Build history of the part. All positions in model axes, mm. Face numbers are marked on the shaded views. A direction names the side the tool comes from. Coordinates: 2 decimals unless noted, no trailing zeros. Loops run counter-clockwise (first coordinate to the right, second up) from the corner with the lowest first, then second, coordinate; pieces in that order, holes last. Notation, with made-up numbers: (-34, 63) - (-1, 63) arc R30 ccw to (-1, 100) - close; hole circle Ø11 at (42.25, 76.5). An arc over 180 degrees is marked (long way). One line per item, written item: value.
```python
from build123d import *

# Parameters (mm, degrees)
SKETCH001_W  = 6
SKETCH001_H  = 6
PAD001_DEPTH = 0.1
FILLET001_R  = 0.3
PAD008_DEPTH = 0.7
FILLET003_R  = 0.29
PAD009_DEPTH = 0.7
FILLET004_R  = 0.29
PAD010_DEPTH = 0.7
FILLET005_R  = 0.29
SKETCH_W     = 6
SKETCH_H     = 6
PAD_DEPTH    = 3.5
FILLET_R     = 0.3
SKETCH004_R  = 0.5
PAD003_DEPTH = 0.6
SKETCH003_R  = 0.5
PAD004_DEPTH = 0.6
SKETCH005_R  = 0.5
PAD002_DEPTH = 0.6
SKETCH002_R  = 0.5
PAD005_DEPTH = 0.6
SKETCH006_R  = 1.75
PAD006_DEPTH = 1.5
FILLET006_R  = 0.1
PAD007_DEPTH = 0.7
FILLET002_R  = 0.29


with BuildPart() as fillet001:
    # Sketch001 → Pad001 (new body)
    with BuildSketch(Plane.XY.offset(3.5)):
        with Locations((3.15, -2.25)):
            Rectangle(SKETCH001_W, SKETCH001_H)
    extrude(amount=PAD001_DEPTH)

    # Fillet001
    fillet001_edges = [fillet001.edges().sort_by_distance(p)[0] for p in [
        (6.15, -5.25, 3.55),
        (0.15, -5.25, 3.55),
        (6.15, 0.75, 3.55),
        (0.15, 0.75, 3.55),
    ]]
    fillet(fillet001_edges, radius=FILLET001_R)


with BuildPart() as fillet003:
    # Sketch008 → Pad008 (new body)
    with BuildSketch(Plane.XZ.offset(0.35)):
        Polygon((-0.15, 1.5), (0.15, 1.5), (0.15, -0.5), (-0.15, -1.5), (0.15, -2.5), (0.15, -3.5), (-0.15, -3.5), (-0.15, -2.5), (-0.45, -1.5), (-0.15, -0.5), align=None)
    extrude(amount=-PAD008_DEPTH)

    # Fillet003
    fillet003_edges = [fillet003.edges().sort_by_distance(p)[0] for p in [
        (-0.15, 0, -2.5),
        (-0.15, 0, -0.5),
        (-0.45, 0, -1.5),
        (-0.15, 0, 1.5),
        (0.15, 0, -0.5),
        (-0.15, 0, -1.5),
        (0.15, 0, -2.5),
    ]]
    fillet(fillet003_edges, radius=FILLET003_R)


with BuildPart() as fillet004:
    # Sketch009 → Pad009 (new body)
    with BuildSketch(Plane.XZ.offset(4.85)):
        Polygon((6.45, 1.5), (6.15, 1.5), (6.15, -0.5), (6.45, -1.5), (6.15, -2.5), (6.15, -3.5), (6.45, -3.5), (6.45, -2.5), (6.75, -1.5), (6.45, -0.5), align=None)
    extrude(amount=-PAD009_DEPTH)

    # Fillet004
    fillet004_edges = [fillet004.edges().sort_by_distance(p)[0] for p in [
        (6.45, -4.5, -2.5),
        (6.45, -4.5, -0.5),
        (6.75, -4.5, -1.5),
        (6.45, -4.5, 1.5),
        (6.15, -4.5, -0.5),
        (6.45, -4.5, -1.5),
        (6.15, -4.5, -2.5),
    ]]
    fillet(fillet004_edges, radius=FILLET004_R)


with BuildPart() as fillet005:
    # Sketch010 → Pad010 (new body)
    with BuildSketch(Plane.XZ.offset(0.35)):
        Polygon((6.45, 1.5), (6.15, 1.5), (6.15, -0.5), (6.45, -1.5), (6.15, -2.5), (6.15, -3.5), (6.45, -3.5), (6.45, -2.5), (6.75, -1.5), (6.45, -0.5), align=None)
    extrude(amount=-PAD010_DEPTH)

    # Fillet005
    fillet005_edges = [fillet005.edges().sort_by_distance(p)[0] for p in [
        (6.45, 0, -2.5),
        (6.45, 0, -0.5),
        (6.75, 0, -1.5),
        (6.45, 0, 1.5),
        (6.15, 0, -0.5),
        (6.45, 0, -1.5),
        (6.15, 0, -2.5),
    ]]
    fillet(fillet005_edges, radius=FILLET005_R)


with BuildPart() as fillet_body:
    # Sketch → Pad (new body)
    with BuildSketch(Plane.XY):
        with Locations((3.15, -2.25)):
            Rectangle(SKETCH_W, SKETCH_H)
    extrude(amount=PAD_DEPTH)

    # Fillet
    fillet_edges = [fillet_body.edges().sort_by_distance(p)[0] for p in [
        (6.15, 0.75, 1.75),
        (6.15, -5.25, 1.75),
        (0.15, -5.25, 1.75),
        (0.15, 0.75, 1.75),
    ]]
    fillet(fillet_edges, radius=FILLET_R)


with BuildPart() as pad003:
    # Pad003 base: copy of Fillet body
    add(fillet_body.part)

    # Sketch004 → Pad003 (new body)
    with BuildSketch(Plane.XY.offset(3.5)):
        with Locations((5.15, -0.25)):
            Circle(SKETCH004_R)
    extrude(amount=PAD003_DEPTH)


with BuildPart() as pad004:
    # Pad004 base: copy of Fillet body
    add(fillet_body.part)

    # Sketch003 → Pad004 (new body)
    with BuildSketch(Plane.XY.offset(3.5)):
        with Locations((5.15, -4.25)):
            Circle(SKETCH003_R)
    extrude(amount=PAD004_DEPTH)


with BuildPart() as pad002:
    # Pad002 base: copy of Fillet body
    add(fillet_body.part)

    # Sketch005 → Pad002 (new body)
    with BuildSketch(Plane.XY.offset(3.5)):
        with Locations((1.15, -0.25)):
            Circle(SKETCH005_R)
    extrude(amount=PAD002_DEPTH)


with BuildPart() as pad005:
    # Pad005 base: copy of Fillet body
    add(fillet_body.part)

    # Sketch002 → Pad005 (new body)
    with BuildSketch(Plane.XY.offset(3.5)):
        with Locations((1.15, -4.25)):
            Circle(SKETCH002_R)
    extrude(amount=PAD005_DEPTH)


with BuildPart() as fillet006:
    # Pad006 base: copy of Fillet body
    add(fillet_body.part)

    # Sketch006 → Pad006 (new body)
    with BuildSketch(Plane.XY.offset(3.5)):
        with Locations((3.15, -2.25)):
            Circle(SKETCH006_R)
    extrude(amount=PAD006_DEPTH)

    # Fillet006
    fillet006_edges = [fillet006.edges().sort_by_distance(p)[0] for p in [
        (1.4, -2.25, 5),
    ]]
    fillet(fillet006_edges, radius=FILLET006_R)


with BuildPart() as obj1:
    # Sketch007 → Pad007 (new body)
    with BuildSketch(Plane.XZ.offset(4.85)):
        Polygon((-0.15, 1.5), (0.15, 1.5), (0.15, -0.5), (-0.15, -1.5), (0.15, -2.5), (0.15, -3.5), (-0.15, -3.5), (-0.15, -2.5), (-0.45, -1.5), (-0.15, -0.5), align=None)
    extrude(amount=-PAD007_DEPTH)

    # Fillet002
    fillet002_edges = [obj1.edges().sort_by_distance(p)[0] for p in [
        (-0.15, -4.5, -2.5),
        (-0.15, -4.5, -0.5),
        (-0.45, -4.5, -1.5),
        (-0.15, -4.5, 1.5),
        (0.15, -4.5, -0.5),
        (-0.15, -4.5, -1.5),
        (0.15, -4.5, -2.5),
    ]]
    fillet(fillet002_edges, radius=FILLET002_R)

    add(fillet001.part)
    add(fillet003.part)
    add(fillet004.part)
    add(fillet005.part)
    add(pad003.part)
    add(pad004.part)
    add(pad002.part)
    add(pad005.part)
    add(fillet006.part)


solid = obj1.part
```
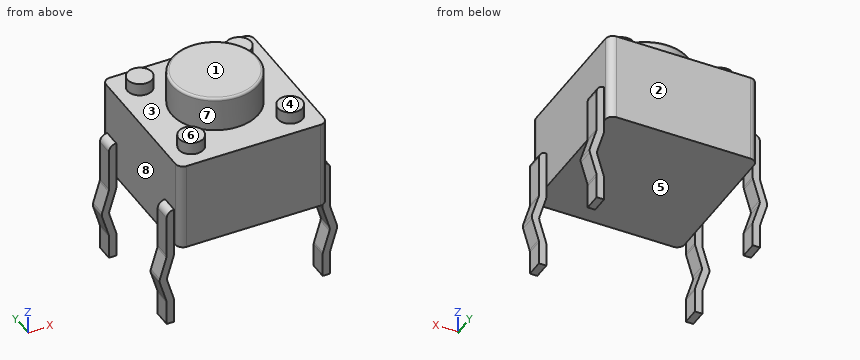
Item 1: Cut at C-C, the plane z = 2.25. Write the cut outline in (x, y).
Check result:
outline: (0.15, -4.95) arc R0.3 ccw to (0.45, -5.25) - (5.85, -5.25) arc R0.3 ccw to (6.15, -4.95) - (6.15, 0.45) arc R0.3 ccw to (5.85, 0.75) - (0.45, 0.75) arc R0.3 ccw to (0.15, 0.45) - close
Item 2: Tool access for the marked faces 4, 5, 6, 7 and 8: list every direction of +Z, -Z, +X, -X, +Y, -Y with a clear straight run to the whole face (end or side of a thin tool).
Check result:
face 4: +Z, +X, -Y
face 5: -Z, +Y, -Y
face 6: +Z, -X, -Y
face 7: +Z
face 8: +Z, -X
Item 3: Cut at D-D, the plane y = -2.25. Write the cut outline in (x, z).
Check result:
outline: (0.15, 0) - (6.15, 0) - (6.15, 3.6) - (4.9, 3.6) - (4.9, 4.9) arc R0.1 ccw to (4.8, 5) - (1.5, 5) arc R0.1 ccw to (1.4, 4.9) - (1.4, 3.6) - (0.15, 3.6) - close
Item 4: Cut at B-B, the plane x = 1.15. Write the cut outline in (y, z), then the cut area to 3 significant figures.
Check result:
outline: (-5.25, 0) - (0.75, 0) - (0.75, 3.6) - (0.25, 3.6) - (0.25, 4.1) - (-0.75, 4.1) - (-0.75, 3.6) - (-3.75, 3.6) - (-3.75, 4.1) - (-4.75, 4.1) - (-4.75, 3.6) - (-5.25, 3.6) - close
area: 22.6 mm^2
Item 5: Pull direction Y, two halves, no side cores. Call the marked faces 1, 2 and 3: released by +Y, released by -Y, zero draft, split by the parting line, or undercut.
Check result:
face 1: zero draft
face 2: released by +Y
face 3: undercut
Item 6: Drop flat-ended pins along their axis: P1, Ø0.8, axis at x = 5, y = -4.5, coming from the +Z side; P2, Ø0.6, axis at y = -4.5, z = 0.5, coming from the -X side; P3, Ø0.5, axis at x = 6.5, z = 0, coming from the -Y side; P4, Ø2, axis at x = 3.5, y = 0, coming from the +Z side. Give the stop position or say it passes through.
Check result:
P1: stops at z = 4.1
P2: stops at x = -0.15
P3: stops at y = -4.85
P4: stops at z = 5
Item 7: Probe probe 1 along X at (y, z) = (-1.05, 0.75); probe 2 along Z at (x, y) = (2, -4.1); probe 3 along Y at (x, z) = (5, 3.75). List the from-to ranges inside material, lowest first. Write a range as from..to.
Check result:
probe 1: x = 0.15..6.15
probe 2: z = 0..3.6
probe 3: y = -4.73..-3.77, -0.73..0.23
Item 8: Cut at A-A, the plane z = -2. Write the cut outline in (x, y).
Check result:
outline: (-0.3, -4.85) - (0, -4.85) - (0, -4.15) - (-0.3, -4.15) - close; (-0.3, -0.35) - (0, -0.35) - (0, 0.35) - (-0.3, 0.35) - close; (6.3, -4.85) - (6.6, -4.85) - (6.6, -4.15) - (6.3, -4.15) - close; (6.3, -0.35) - (6.6, -0.35) - (6.6, 0.35) - (6.3, 0.35) - close
